Input: dimensioned drawing with shaded views. Units: mm. Origin: part minimum x, y, z. Give positions to 0.01 mm unless a question says otherwise; leave off trailing zeros. Loops run counter-clockwise (first coordinate to the right, second up) from the corner with the lowest first, then second, coordinate; pieces in that order, holes last. Notation, with made-up numbers: M -38,-13 L -14,-13 A17 ccw -14,14 Z; hole C 45,-5 d3. An arc over 180 degrees is marked long. Answer in a Markdown table with one row per item.
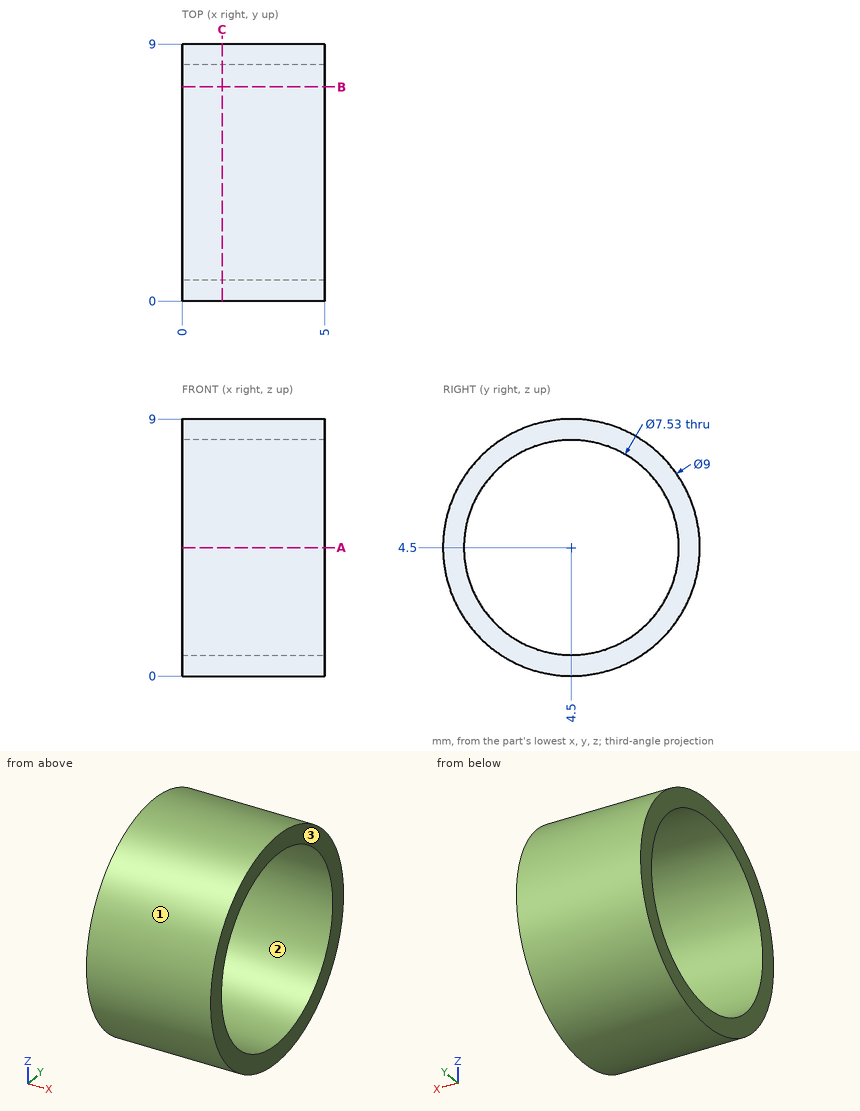
Q1. Mould query, pull axis Z, two halves, no side actions, for the marked faces 1, 2 and 3. Classes: +Z half, -Z half, draft (parallel to the pull), parting line (faces both ways), or undercut.
Values follow:
| item | result |
|---|---|
| face 1 | parting line |
| face 2 | undercut |
| face 3 | draft |
Q2. Ray query, probe 1 along Y at (x, z) = (3.25, 4.5) (3 decimals); probe 2 along Y at (x, z) = (1.7, 5); probe 3 along Z at (x, y) = (2.65, 3). Return the intervals inside material, ascending. Write a range as from..to.
Values follow:
| item | result |
|---|---|
| probe 1 | 0..0.735, 8.265..9 |
| probe 2 | 0.03..0.77, 8.23..8.97 |
| probe 3 | 0.26..1.05, 7.95..8.74 |
Q3. Section query C-C (x = 1.4). Output: boundary loops of the cut face in (y, z) (3 decimals), plus the area to 3 significant figures.
Values follow:
| item | result |
|---|---|
| outline | C 4.5,4.5 d9; hole C 4.5,4.5 d7.53 |
| area | 19.1 mm^2 |
Q4. Section query A-A (z = 4.5). Output: boundary loops of the cut face in (x, y) (3 decimals), plus the area to 3 significant figures.
Values follow:
| item | result |
|---|---|
| outline | M 0,0 L 5,0 L 5,0.735 L 0,0.735 Z; M 0,8.265 L 5,8.265 L 5,9 L 0,9 Z |
| area | 7.35 mm^2 |
Q5. Section query B-B (y = 7.5). Output: boundary loops of the cut face in (x, z), plus the area to 3 significant figures.
Values follow:
| item | result |
|---|---|
| outline | M 0,1.15 L 5,1.15 L 5,2.23 L 0,2.23 Z; M 0,6.77 L 5,6.77 L 5,7.85 L 0,7.85 Z |
| area | 10.8 mm^2 |
Q6. Contact query for flat-ended pins moving along their axis: pin 1 Ø1 at (x, y) = (3.5, 6) entering from +Z; pin 2 Ø1.5 at (x, z) = (1.5, 6.5) entering from -Y; pin 3 Ø1.5 at (x, z) = (2, 3) entering from -Y. Output: stop coordinate, or through.
Values follow:
| item | result |
|---|---|
| pin 1 | z = 8.89 |
| pin 2 | y = 0.18 |
| pin 3 | y = 0.06 |
